Autodesk Fusion 360 part; units mm, degrees
sketch "Esboço1" plane through (0, 0, 0) normal (0, 0, 1) x (1, 0, 0) in component "Case"
sketch "Esboço1 (2)" plane through (0, 0, 0) normal (0, 0, 1) x (1, 0, 0) in component "Component"
  line L0 (-33.5931, -33.1775) -> (13.2718, -33.1775)
  line L1 (13.2718, -33.1775) -> (13.2718, 52.9754)
  line L2 (13.2718, 52.9754) -> (-33.5931, 52.9754)
  line L3 (-33.5931, 52.9754) -> (-33.5931, -33.1775)
  line L4 (-40, 60) -> (20, 60)
  line L5 (20, 60) -> (20, -40)
  line L6 (20, -40) -> (-40, -40)
  line L7 (-40, -40) -> (-40, 60)
  circle A0 centre (-35, -35) radius 1.7
  circle A1 centre (15, -35) radius 1.7
  circle A2 centre (-35, 55) radius 1.7
  circle A3 centre (15, 55) radius 1.7
  dimension "d1" = 86.1529
  dimension "d2" = 46.8649
  dimension "d5" = 5
  dimension "d6" = 5
  dimension "d7" = 5
  dimension "d8" = 5
  dimension "d9" = 5
  dimension "d10" = 5
  dimension "d11" = 5
  dimension "d12" = 5
  dimension "d13" = 60
  dimension "d14" = 100
extrude "Extrusão1" add sketch "Esboço1 (2)" along normal blind 9.9 contours A0 | A1 | A2 | A3 makes body 1 at (-35.7756, -33.4872, 6.6) makes body 2 at (-35.7756, 56.5128, 6.6) makes body 3 at (16.5665, -34.3397, 6.6) makes body 4 at (16.5665, 55.6603, 6.6) in component "Component"
extrude "Extrusão2" add sketch "Esboço1 (2)" along normal blind 13 bodies 1 2 3 4 in component "Component"
extrude "Extrusão3" add sketch "Esboço1 (2)" along normal blind 3 contours L0 L1 L2 L3 bodies 1 in component "Component"
sketch "Esboço2" plane through (0, 0, 13) normal (0, 0, 1) x (-1, 0, 0) in component "Component"
  circle A0 centre (-15, -55) radius 1.7
  line L0 (33.5931, 33.1775) -> (33.5931, -52.9754)
  line L1 (33.5931, -52.9754) -> (-13.2718, -52.9754)
  line L2 (-13.2718, -52.9754) -> (-13.2718, 33.1775)
  line L3 (-13.2718, 33.1775) -> (33.5931, 33.1775)
  circle A1 centre (35, 35) radius 1.7
  circle A2 centre (-15, 35) radius 1.7
  circle A3 centre (35, -55) radius 1.7
  line L4 (40, 40) -> (-20, 40)
  line L5 (-20, 40) -> (-20, -60)
  line L6 (-20, -60) -> (40, -60)
  line L7 (40, -60) -> (40, 40)
  line L8 (15.0931, -60) -> (6.2282, -60)
  line L9 (6.2282, -60) -> (6.2282, -52.9754)
  line L10 (6.2282, -52.9754) -> (15.0931, -52.9754)
  line L11 (15.0931, -52.9754) -> (15.0931, -60)
  dimension "d21" = 18.5
  dimension "d22" = 19.5
extrude "Extrusão4" cut sketch "Esboço2" against normal blind 7.5 contours L1 L6 L8 L9 L10 L11 bodies 1 in component "Component"
fillet "Arredondamento1" radius 5 1 edges at (20, -40, 6.5) on bodies 1 in component "Component"
fillet "Arredondamento2" radius 5 1 edges at (-40, -40, 6.5) on bodies 1 in component "Component"
fillet "Arredondamento3" radius 5 1 edges at (-40, 60, 6.5) on bodies 1 in component "Component"
fillet "Arredondamento4" radius 5 1 edges at (20, 60, 6.5) on bodies 1 in component "Component"
component "Case" placed x (1, 0, 0) y (0, 1, 0) z (0, 0, 1) at (0, 0, 0)
component "Component" placed x (1, 0, 0) y (0, 1, 0) z (0, 0, 1) at (0, 0, 0) in component "Case"
Design review of the part built by this model. Coordinates are the model's own, in mm. A direction names the side the tool comes from. Coordinates: 2 decimals unless noted, no trailing zeros. Order: outer loops, then holes, each group sorted by start corner. A loop starts at its lowest first (then second) coordinate and runs counter-clockwise, first axis right, second up.
1) For faces 5 (the flat face through (-10, -40, 6)), 6 (the flat face through (15, -35, 9.9)), 7 (the flat face through (-11, 56, 5.5)), list the 3-axis set-ups (+Z, -Z, +X, -X, +Y, -Y) from which the entire face can be reached by the end or side of a thin tool; tool diameter is ignored.
2) Clearance check with flat-ended pins moving along their axes: pin 1 (4.5 mm diameter, centred on x = 15, y = 55, fed in from +Z); pin 2 (3.5 mm diameter, centred on y = 57.5, z = 10, fed in from +X); pin 3 (6 mm diameter, centred on x = -27.5, y = -23.5, fed in from +Z); pin 4 (1.7 mm diameter, centred on x = -35.5, y = 55, fed in from +Z). State where each tip first meets the part, or that it passes through.
3) Take a section at C-C, the plane y = -24. Give the boundary of the cut face in (x, z), and give its area (3 significant figures).
4) Take a section at A-A, the plane z = 4.25. Give the boundary of the cut face in (x, y).
5) Take a section at B-B, the plane x = -18.5. Give the boundary of the cut face in (y, z), and give its area (3 significant figures).
6) Mouldability with a two-part tool opening along Y and no side actions: class faces 1 (the cylindrical face through (-39, -38, 7)), 2 (the flat face through (-10, -33.178, 8)), 3 (the flat face through (-6.228, 57, 9)), 4 (the flat face through (-35, -35, 9.9)) as +Y half, -Y half, draft (parallel to the pull), parting line (faces both ways), or undercut.
7) Wall thickness on line 1 along Y through (x, z) = (-35, 11.45); line 2 along X through (y, z) = (46, 10); line 3 along Y through (x, z) = (-22.5, 10): over which ranges is each line inside the solid? List them lowest first.
Returned:
1. face 5: +Z, -Z, +X, -X, -Y
1. face 6: +Z
1. face 7: +Z, +Y
2. pin 1: stops at z = 13
2. pin 2: stops at x = 19.94
2. pin 3: stops at z = 3
2. pin 4: stops at z = 9.9
3. outline: (-40, 0) - (20, 0) - (20, 13) - (13.27, 13) - (13.27, 3) - (-33.59, 3) - (-33.59, 13) - (-40, 13) - close
3. area: 311 mm2
4. outline: (-40, -35) arc R5 ccw to (-35, -40) - (15, -40) arc R5 ccw to (20, -35) - (20, 55) arc R5 ccw to (15, 60) - (-35, 60) arc R5 ccw to (-40, 55) - close; hole (-33.59, -33.18) - (13.27, -33.18) - (13.27, 52.98) - (-33.59, 52.98) - close
5. outline: (-40, 0) - (60, 0) - (60, 13) - (52.98, 13) - (52.98, 3) - (-33.18, 3) - (-33.18, 13) - (-40, 13) - close
5. area: 438 mm2
6. face 1: -Y half
6. face 2: undercut
6. face 3: draft
6. face 4: undercut
7. line 1: y = -40 to -36.7, -33.3 to 53.3, 56.7 to 60
7. line 2: x = -40 to -33.59, 13.27 to 20
7. line 3: y = -40 to -33.18, 52.98 to 60
